Input: part model. Units: mm. Frame: model coordinates. Round coordinates to 2 decimals unless told otherwise and drop trailing zeros. Loops run counter-clockwise (first coordinate to the right, second up) from the corner with the lowest first, then second, coordinate; pieces in that order, holes last. Notation, with made-up numbers: (-4.5, 72) - (14.5, 72) arc R25 cw to (14.5, 97) - close; hole circle Ø6 at (-17, 22). An arc over 180 degrees is marked (long way). Use CSV: the item, a comma, the result in double quotes. Start each with the question number.
1. Cut plane B-B (x = 17.5). Return loops of the section in (y, z).
2. Material intervals for probe 1 along Y at (x, z) = (11, 1.85); probe 2 along Y at (x, z) = (-8, 2.6); probe 3 along X at (y, z) = (-26.5, 0.9), sorted ascending. Write a range as from..to.
3. Cut plane C-C (x = -13). Return loops of the section in (y, z).
4. Cut plane D-D (z = 1.8). Give the number of separate pieces and of enclosed holes in the cut face, and give its area (3 significant figures).
5. Cut plane A-A (y = -11.5). Return loops of the section in (x, z).
6. Pin query (flat end, axial travel): P1, Ø0.9, axis at y = -3.5, z = 2, coming from the +X side. Return the tip coordinate at first contact, or that it passes through.
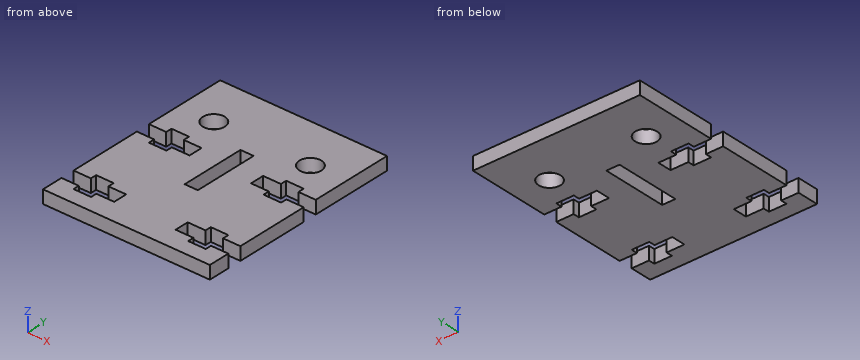
```python
from build123d import *

# Parameters (mm, degrees)
SKETCH1_W           = 38
SKETCH1_H           = 47
BOSS_EXTRUDE1_DEPTH = 3
SKETCH2_R           = 2.5
CUT_EXTRUDE1_DEPTH  = 3
CUT_EXTRUDE2_DEPTH  = 3
SKETCH4_W           = 3
SKETCH4_H           = 14.8
CUT_EXTRUDE3_DEPTH  = 10


with BuildPart() as part:
    # Sketch1 → Boss-Extrude1 (new body)
    with BuildSketch(Plane.XY):
        with Locations((0, -6.895095368)):
            Rectangle(SKETCH1_W, SKETCH1_H)
    extrude(amount=BOSS_EXTRUDE1_DEPTH)

    # Sketch2 → Cut-Extrude1 (cut)
    with BuildSketch(Plane.XY.offset(3)):
        with Locations((-11, 5.604904632)):
            Circle(SKETCH2_R)
        with Locations(Location((11, 5.604904632, 0), (0, 0, 180))):
            Circle(SKETCH2_R)
    extrude(amount=-CUT_EXTRUDE1_DEPTH, mode=Mode.SUBTRACT)

    # Sketch3 → Cut-Extrude2 (cut)
    with BuildSketch(Plane.XY.offset(3)):
        Polygon((-7, -5.495095368), (-11.059072882, -5.495095368), (-11.059072882, -6.895095368), (-15.059072882, -6.895095368), (-15.059072882, -5.495095368), (-19, -5.495095368), (-19, -2.295095368), (-15.059072882, -2.295095368), (-15.059072882, -0.895095368), (-11.059072882, -0.895095368), (-11.059072882, -2.295095368), (-7, -2.295095368), align=None)
        Polygon((7, -5.495095368), (11.059072882, -5.495095368), (11.059072882, -6.895095368), (15.059072882, -6.895095368), (15.059072882, -5.495095368), (19, -5.495095368), (19, -2.295095368), (15.059072882, -2.295095368), (15.059072882, -0.895095368), (11.059072882, -0.895095368), (11.059072882, -2.295095368), (7, -2.295095368), align=None)
        Polygon((-7, -25.495095368), (-7, -22.295095368), (-11.059072882, -22.295095368), (-11.059072882, -20.895095368), (-15.059072882, -20.895095368), (-15.059072882, -22.295095368), (-19, -22.295095368), (-19, -25.495095368), (-15.059072882, -25.495095368), (-15.059072882, -26.895095368), (-11.059072882, -26.895095368), (-11.059072882, -25.495095368), align=None)
        Polygon((7, -25.495095368), (11.059072882, -25.495095368), (11.059072882, -26.895095368), (15.059072882, -26.895095368), (15.059072882, -25.495095368), (19, -25.495095368), (19, -22.295095368), (15.059072882, -22.295095368), (15.059072882, -20.895095368), (11.059072882, -20.895095368), (11.059072882, -22.295095368), (7, -22.295095368), align=None)
    extrude(amount=-CUT_EXTRUDE2_DEPTH, mode=Mode.SUBTRACT)

    # Sketch4 → Cut-Extrude3 (cut)
    with BuildSketch(Plane.XY.offset(3)):
        with Locations((0, -5.795095368)):
            Rectangle(SKETCH4_W, SKETCH4_H)
    extrude(amount=-CUT_EXTRUDE3_DEPTH, mode=Mode.SUBTRACT)


solid = part.part
```
Established:
1,outline,"(-30.4, 0) - (-25.5, 0) - (-25.5, 3) - (-30.4, 3) - close; (-22.3, 0) - (-5.5, 0) - (-5.5, 3) - (-22.3, 3) - close; (-2.3, 0) - (16.6, 0) - (16.6, 3) - (-2.3, 3) - close"
2,probe 1,"y = -30.4..-25.5, -22.3..-5.5, -2.3..3.1, 8.1..16.6"
2,probe 2,"y = -30.4..-25.5, -22.3..-5.5, -2.3..16.6"
2,probe 3,"x = -19..-15.06, -11.06..11.06, 15.06..19"
3,outline,"(-30.4, 0) - (-26.9, 0) - (-26.9, 3) - (-30.4, 3) - close; (-20.9, 0) - (-6.9, 0) - (-6.9, 3) - (-20.9, 3) - close; (-0.9, 0) - (4.1, 0) - (4.1, 3) - (-0.9, 3) - close; (7.1, 0) - (16.6, 0) - (16.6, 3) - (7.1, 3) - close"
4,separate pieces,"1"
4,enclosed holes,"3"
4,area,"1,500 mm2"
5,outline,"(-19, 0) - (-1.5, 0) - (-1.5, 3) - (-19, 3) - close; (1.5, 0) - (19, 0) - (19, 3) - (1.5, 3) - close"
6,P1,"stops at x = 7"
